The listing builds one solid part. Answer for the finished solid, in the listing's coordinates (mm). A direction names the side the tool comes from. Give positions to 0.01 mm unless a question says otherwise; leave off trailing zeros. Write each loop counter-clockwise with the first axis right and the second up, starting at its lowest first coordinate (ties: lowest second). Pieces come first, ordered by that corner, then holes. Notation, with made-up numbers: (68, -33.75) - (90, -33.75) arc R17 ccw to (90, -14.75) - close; hole circle Ø6 at (-30, -39.75). An arc over 180 degrees is marked (long way). Write each question's results on one line, items separated by ' | '. Start each with the question number.
Q1. Section C-C (z = -6) is taken. Determine the outline of the cut face in (x, y), plus the area to 3 significant figures.
Q2. For a pull along Z with two mould halves and no side action, classify faces 6 (the face through (-39, -44, 7)), 7 (the face through (20, -43, -10)), 8 (the face through (-40, -44, 6)), 9 (the face through (3.591, -48, -1)) as pulls with the +Z half, pulls with the -Z half, needs draft (parallel to the pull), parting line crosses it, or undercut.
Q3. Find the intervals of material crossed by probe 1 along Z at (x, y) = (-37.5, -9); probe 2 along Z at (x, y) = (24, -35); probe 3 along X at (y, z) = (-50, -0.75), in increasing order.
Q4. Section A-A (x = -10.5) is taken. Determine the outline of the cut face in (y, z), plus the area to 3 significant figures.
Q5. Flat-ended cylindrical pins translate along their axes: pin 1 Ø10 at (x, y) = (-26, -69) entering from +Z; pin 2 Ø6.5 at (x, y) = (40, -26) entering from -Z; pin 3 Ø4.5 at (x, z) = (0, -8.5) entering from +Y. Find the tip coordinate at first contact, or state that the pin passes through.
Q6. For faces 1 (the face through (27, -43, -6)), 2 (the face through (-21.409, -50, -1)), 3 (the face through (-10, -88, -6)), 4 (the face through (10, -44, 0)), 5 (the face through (28, -43, -6)), determine the directions among +Z, -Z, +X, -X, +Y, -Y from which every point of the face is accessible in a straight line to the end or side of a thin tool.
Q7. Section D-D (y = -10.5) is taken. Determine the outline of the cut face in (x, z), plus the area to 3 significant figures.
Q8. Section B-B (y = -40) is taken. Determine the outline of the cut face in (x, z).
```python
from build123d import *

# Parameters (mm, degrees)
F1_DEPTH = 88
F3_DEPTH = 1
F4_DEPTH = 88
F6_DEPTH = 1
F8_DEPTH = 2


with BuildPart() as f1:
    # F0 (on Front) → F1 (new body)
    with BuildSketch(Plane.XZ):
        Polygon((43, 0), (0, 0), (-43, 0), (-43, 6), (-37, 6), (-37, 7), (-44, 7), (-44, -1), (0, -1), (28, -1), (44, -1), (44, 7), (37, 7), (37, 6), (43, 6), align=None)
    extrude(amount=F1_DEPTH)

    # F2 (on face) → F3 (join)
    with BuildSketch(Plane(origin=(0, 0, 0), x_dir=(-1, 0, 0), z_dir=(0, 1, 0))):
        Polygon((37, 7), (-37, 7), (-37, 6), (-43, 6), (-43, 0), (43, 0), (43, 6), (37, 6), align=None)
    extrude(amount=-F3_DEPTH)

    # F0 (on Front) → F4 (join)
    with BuildSketch(Plane.XZ):
        Polygon((0, -1), (-44, -1), (-44, -11), (-29, -11), (-29, -10), (-43, -10), (-43, -2), (0, -2), (27, -2), (27, -10), (13, -10), (13, -11), (28, -11), (28, -2), (28, -1), align=None)
    extrude(amount=F4_DEPTH)

    # F5 (on face) → F6 (join)
    with BuildSketch(Plane.XZ.offset(88)):
        Polygon((-29, -10), (-29, -11), (13, -11), (13, -10), (27, -10), (27, -2), (-43, -2), (-43, -10), align=None)
    extrude(amount=-F6_DEPTH)

    # F7 (on Top) → F8 (cut)
    with BuildSketch(Plane.XY):
        Polygon((-21.4086160213, -63.8053458929), (3.5913839787, -63.8053458929), (3.5913839787, -31.8053458929), (-17.4086160213, -31.8053458929), (-21.4086160213, -35.8053458929), align=None)
    extrude(amount=-F8_DEPTH, mode=Mode.SUBTRACT)


solid = f1.part
```
Answers below:
1) outline: (-44, -88) - (28, -88) - (28, 0) - (27, 0) - (27, -87) - (-43, -87) - (-43, 0) - (-44, 0) - close | area: 246 mm2
2) face 6: pulls with the +Z half | face 7: undercut | face 8: undercut | face 9: needs draft
3) probe 1: z = -11 to -10, -2 to 0, 6 to 7 | probe 2: z = -11 to -10, -2 to 0 | probe 3: x = -44 to -21.41, 3.59 to 44
4) outline: (-88, -11) - (-87, -11) - (-87, -2) - (-63.81, -2) - (-63.81, 0) - (-88, 0) - close; (-31.81, -2) - (0, -2) - (0, 7) - (-1, 7) - (-1, 0) - (-31.81, 0) - close | area: 128 mm2
5) pin 1: stops at z = 0 | pin 2: stops at z = -1 | pin 3: stops at y = -87
6) face 1: +Y | face 2: +Z, -Z | face 3: +Z, -Z, +X, -X, -Y | face 4: -Y | face 5: -Z, +X, +Y, -Y
7) outline: (-44, -11) - (-29, -11) - (-29, -10) - (-43, -10) - (-43, -2) - (27, -2) - (27, -10) - (13, -10) - (13, -11) - (28, -11) - (28, -1) - (44, -1) - (44, 7) - (37, 7) - (37, 6) - (43, 6) - (43, 0) - (-43, 0) - (-43, 6) - (-37, 6) - (-37, 7) - (-44, 7) - close | area: 232 mm2
8) outline: (-44, -11) - (-29, -11) - (-29, -10) - (-43, -10) - (-43, -2) - (-21.41, -2) - (-21.41, 0) - (-43, 0) - (-43, 6) - (-37, 6) - (-37, 7) - (-44, 7) - close; (3.59, -2) - (27, -2) - (27, -10) - (13, -10) - (13, -11) - (28, -11) - (28, -1) - (44, -1) - (44, 7) - (37, 7) - (37, 6) - (43, 6) - (43, 0) - (3.59, 0) - close
